from build123d import *

# Parameters (mm, degrees)
SKETCH1_R           = 1.5
SKETCH1_R_2         = 1.65
BOSS_EXTRUDE1_DEPTH = 6.35
FILLET2_R           = 10
SKETCH2_R           = 0.5
CUT_EXTRUDE1_DEPTH  = 73.122135992


with BuildPart() as part:
    # Sketch1 → Boss-Extrude1 (new body)
    with BuildSketch(Plane.XY):
        with BuildLine():
            Line((24.062500008, -40.5), (24.062500008, 40.5))
            Line((24.062500008, 40.5), (24.062500008, 44.73964789))
            ThreePointArc((24.062500008, 44.73964789), (0, -50.8), (-24.062500008, 44.73964789))
            Line((-24.062500008, 44.73964789), (-24.062500008, 40.5))
            Line((-24.062500008, 40.5), (-24.062500008, -40.5))
            Line((-24.062500008, -40.5), (24.062500008, -40.5))
        make_face()
        with Locations((-45.72, 0)):
            Circle(SKETCH1_R, mode=Mode.SUBTRACT)
        with Locations((45.72, 0)):
            Circle(SKETCH1_R, mode=Mode.SUBTRACT)
        with Locations((-39.594681461, 22.86)):
            Circle(SKETCH1_R_2, mode=Mode.SUBTRACT)
        with Locations((39.594681461, 22.86)):
            Circle(SKETCH1_R_2, mode=Mode.SUBTRACT)
        with Locations((39.594681461, -22.86)):
            Circle(SKETCH1_R_2, mode=Mode.SUBTRACT)
        with Locations((0, -45.72)):
            Circle(SKETCH1_R_2, mode=Mode.SUBTRACT)
        with Locations((-39.594681461, -22.86)):
            Circle(SKETCH1_R_2, mode=Mode.SUBTRACT)
    extrude(amount=BOSS_EXTRUDE1_DEPTH)

    # Fillet2
    fillet2_edges = [part.edges().sort_by_distance(p)[0] for p in [
        (24.062500008, 44.73964789, 3.175),
        (-24.062500008, 44.73964789, 3.175),
    ]]
    fillet(fillet2_edges, radius=FILLET2_R)

    # Sketch2 → Cut-Extrude1 (cut, through all)
    with BuildSketch(Plane.XY.offset(6.35)):
        with Locations((-24.062500008, -40.5)):
            Circle(SKETCH2_R)
        with Locations((24.062500008, -40.5)):
            Circle(SKETCH2_R)
    extrude(amount=-CUT_EXTRUDE1_DEPTH, mode=Mode.SUBTRACT)


solid = part.part
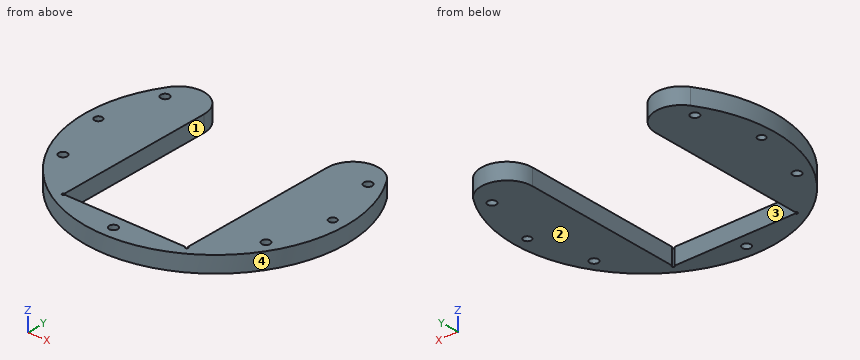
Source: CAD feature listing. Evaluate the final solid. Frame: model axes, mm. Face numbers are marked on the shaded views. Give positions to 0.01 mm unless a question says otherwise; leave off trailing zeros. Write each loop counter-clockwise with the first axis right and the second up, starting at its lowest first coordinate (ties: lowest second). Pieces come first, ordered by that corner, then holes. Notation, with made-up numbers: M 82,-32.75 L 93,-32.75 A18 cw 93,-7.75 Z; hole C 36,23.5 d5. An arc over 180 degrees is marked long. Answer as a JSON object with one key per item and string values.
Q1. Ray query, line 1 along Y through (x, z) = (0, 2.75); line 2 along X through (y, z) = (18, 5); line 3 along Y through (x, z) = (45.72, 4.25). Return the intervals inside material, ascending.
Geometry check:
{"line 1": "y = -50.8 to -47.37, -44.07 to -40.5", "line 2": "x = -47.5 to -24.06, 24.06 to 47.5", "line 3": "y = -22.14 to -1.5, 1.5 to 22.14"}
Q2. Cut plane B-B, the plane z = 2.25. Return the cut outline in (x, y).
Geometry check:
{"outline": "M -42.41,27.96 A50.8 ccw long 42.41,27.96 A10 ccw 24.06,22.46 L 24.06,-40 A0.5 cw long 23.56,-40.5 L -23.56,-40.5 A0.5 cw long -24.06,-40 L -24.06,22.46 A10 ccw Z; hole C -45.72,0 d3; hole C -39.59,-22.86 d3.3; hole C -39.59,22.86 d3.3; hole C 0,-45.72 d3.3; hole C 39.59,-22.86 d3.3; hole C 39.59,22.86 d3.3; hole C 45.72,0 d3"}
Q3. Mould query, pull axis X, two halves, no side actions, for the marked faces 1, 2, 3 and 4. Classes: +X half, -X half, draft (parallel to the pull), parting line (faces both ways), or undercut.
Geometry check:
{"face 1": "undercut", "face 2": "draft", "face 3": "undercut", "face 4": "parting line"}
Q4. Cut plane A-A, the plane y = 0. Return the cut outline in (x, z).
Geometry check:
{"outline": "M -50.8,0 L -47.22,0 L -47.22,6.35 L -50.8,6.35 Z; M -44.22,0 L -24.06,0 L -24.06,6.35 L -44.22,6.35 Z; M 24.06,0 L 44.22,0 L 44.22,6.35 L 24.06,6.35 Z; M 47.22,0 L 50.8,0 L 50.8,6.35 L 47.22,6.35 Z"}
Q5. Cut plane C-C, the plane y = 11.5. Return the cut outline in (x, z).
Geometry check:
{"outline": "M -49.48,0 L -24.06,0 L -24.06,6.35 L -49.48,6.35 Z; M 24.06,0 L 49.48,0 L 49.48,6.35 L 24.06,6.35 Z"}
Q6. Cut plane D-D, the plane x = 45.72. Return the cut outline in (y, z), then the cut area to 3 significant figures.
Geometry check:
{"outline": "M -22.14,0 L -1.5,0 L -1.5,6.35 L -22.14,6.35 Z; M 1.5,0 L 22.14,0 L 22.14,6.35 L 1.5,6.35 Z", "area": "262 mm^2"}
Q7. Contact query for flat-ended pins moving along their axis: P1, Ø1.9, axis at x = 7, z = 3.5, coming from the +Y side; P2, Ø3.5, axis at x = 45.72, y = 0, coming from the -Z side; P3, Ø1.8, axis at x = -45.72, y = 0, coming from the +Z side; P4, Ø3, axis at y = -10.5, z = 3.5, coming from the -X side. Output: stop coordinate, or through.
Geometry check:
{"P1": "stops at y = -40.5", "P2": "stops at z = 0", "P3": "passes through", "P4": "stops at x = -50"}
